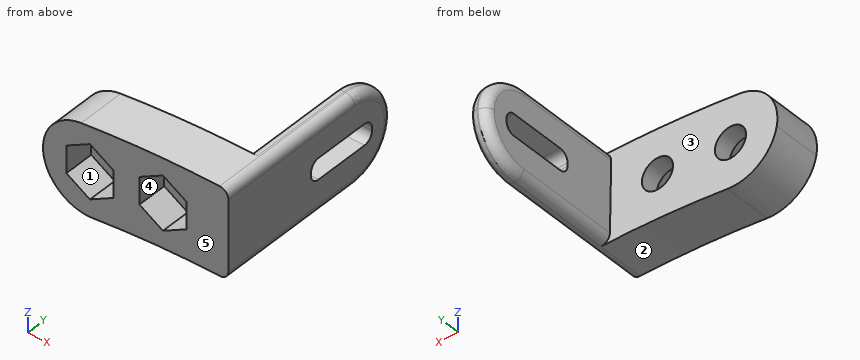
from build123d import *

# Parameters (mm, degrees)
EXTRUDE_1_DEPTH     = 8
EXTRUDE_2_DEPTH     = 25
HOLE_WIZARD_M5_1_D  = 5.3
FILLET_1_R          = 7.5
FILLET_2_DEPTH      = 8
SKETCH_5_W          = 3.5999999999999943
SKETCH_5_H          = 12.29999999986595
FILLET_3_R          = 1.5
FILLET_4_R          = 1.5
CUT_EXTRUDE_1_DEPTH = 5


with BuildPart() as part:
    # 草图1 → 凸台-拉伸1 (new body)
    with BuildSketch(Plane(origin=(0, 0, 0), x_dir=(1, 0, 0), z_dir=(0, 1, 0))):
        with BuildLine():
            Line((2.098e-14, -189), (1.932e-14, -174.00000000000003))
            ThreePointArc((2.28618e-12, -174.00000000000003), (-15.165099238093463, -173.33787746796366), (-30.214782914050144, -171.35654902412347))
            Line((-30.214782914045937, -171.35654902412418), (-32.8195055790499, -186.12866531930732))
            ThreePointArc((-32.81950557905, -186.12866531930732), (-16.472435379307413, -188.28079793933995), (-3.472e-14, -189.00000000000003))
        make_face()
    extrude(amount=EXTRUDE_1_DEPTH)

    # 草图4 → 凸台-拉伸2 (add)
    with BuildSketch(Plane(origin=(0, 8, 0), x_dir=(1, 0, 0), z_dir=(0, 1, 0))):
        with BuildLine():
            Line((2.082e-14, -189), (1.916e-14, -174))
            ThreePointArc((-3.196e-14, -174.00000000000003), (-1.5184171767173116, -173.99337461316583), (-3.0367187200877925, -173.9734989572121))
            Line((-3.036718720087315, -173.97349895721206), (-3.298504816646567, -188.97121438455795))
            ThreePointArc((-3.2985048166465822, -188.971214384558), (-1.6493152091926062, -188.99280345912842), (-3.472e-14, -189.00000000000006))
        make_face()
    extrude(amount=EXTRUDE_2_DEPTH)

    # M5 间隙孔1 (through all)
    with Locations(Plane(origin=(0, 8, 0), x_dir=(1, 0, 0), z_dir=(0, 1, 0))):
        with Locations((-23.608051681, -179.958078162), (-11.163314825, -181.156370029)):
            Hole(HOLE_WIZARD_M5_1_D / 2)

    # 圆角1
    # the kernel refuses this fillet: 7.5 mm, written as the material it takes off along each edge
    with BuildSketch(Plane(origin=(1.47232e-12, 33, -1.0760459e-10), x_dir=(0.10755019962978496, 0, 0.9941996552803635), z_dir=(0.9941996552803635, 0, -0.10755019962978496))) as fillet_1_piece_1:
        with BuildLine():
            CenterArc((174.00000000010766 + FILLET_1_R, FILLET_1_R), FILLET_1_R, 180, 89.99999999999977)
            Line((174.00000000010766 + FILLET_1_R, 0), (174.00000000010766, 0))
            Line((174.00000000010766, 0), (174.00000000010766, FILLET_1_R))
        make_face()
    fillet_1_piece_1_solid = revolve(axis=Axis((1.47232e-12, 33, -1.0760459e-10), (0, -1, 0)), revolution_arc=13.348228955549553, mode=Mode.PRIVATE)
    with BuildSketch(Plane(origin=(2.05469e-12, 33, -2.9481839e-10), x_dir=(-0.11639521392683701, 0, 0.9932029773288671), z_dir=(-0.9932029773288671, 0, -0.11639521392683701))) as fillet_1_piece_2:
        with BuildLine():
            CenterArc((189.0000000002949 - FILLET_1_R, -FILLET_1_R), FILLET_1_R, 0, 89.99999999999957)
            Line((189.0000000002949 - FILLET_1_R, 0), (189.0000000002949, 0))
            Line((189.0000000002949, 0), (189.00000000029488, -FILLET_1_R))
        make_face()
    fillet_1_piece_2_solid = revolve(axis=Axis((2.05469e-12, 33, -2.9481839e-10), (0, 1, 0)), revolution_arc=12.368210784462358, mode=Mode.PRIVATE)
    add([fillet_1_piece_1_solid, fillet_1_piece_2_solid], mode=Mode.SUBTRACT)

    # 圆角2: read off the stored shape, not the designer's step
    # 圆角2 outline → 圆角2 (cut)
    with BuildSketch(Plane(origin=(0, 0, 0), x_dir=(1, 0, 0), z_dir=(0, 1, 0))):
        with BuildLine():
            ThreePointArc((-32.819505579, -186.128665319), (-28.966041771, -186.767150281), (-25.100206236, -187.325864863))
            add(Edge.make_bspline(
                [(-25.100206236, -187.325864863), (-27.006863278382305, -187.07038767754574), (-29.132080374521447, -186.17341393049847), (-31.048536919413714, -184.35464406978926), (-32.02623112721157, -181.62978297542463), (-31.490224503, -178.589937725)],
                knots=[0, 0, 0, 0, 0, 0, 0.5103349834155644, 0.5103349834155644, 0.5103349834155644, 0.5103349834155644, 0.5103349834155644, 0.5103349834155644], degree=5, weights=[1, 0.7958660065557144, 0.6438203721908997, 0.5438630969055563, 0.4959941806996843, 0.5002136235732837]))
            Line((-31.490224503, -178.589937725), (-32.819505579, -186.128665319))
        make_face()
        with BuildLine():
            Line((-30.214782914, -171.356549024), (-31.490224503, -178.589937725))
            add(Edge.make_bspline(
                [(-31.490224503, -178.589937725), (-30.984360135627078, -175.72103774319677), (-29.29551148466263, -173.58668082656104), (-27.075163325391554, -172.48015181385665), (-24.918748626576246, -172.21612345785414), (-23.108126376, -172.458732732)],
                knots=[0.5103349834155644, 0.5103349834155644, 0.5103349834155644, 0.5103349834155644, 0.5103349834155644, 0.5103349834155644, 1, 1, 1, 1, 1, 1], degree=5, weights=[0.5002136235732837, 0.5042621674352976, 0.5562650770089762, 0.6562223522943196, 0.8041339932913276, 1]))
            ThreePointArc((-23.108126376, -172.458732732), (-26.667149567, -171.944360576), (-30.214782914, -171.356549024))
        make_face()
    extrude(amount=FILLET_2_DEPTH, mode=Mode.SUBTRACT)

    # 草图5 → 切除-旋转1 (revolve, cut)
    with BuildSketch(Plane(origin=(0, 0, 0), x_dir=(-0.01745240643728342, 0, 0.9998476951563913), z_dir=(-0.9998476951563913, 0, -0.01745240643728342))):
        with Locations((181.5, 22.85000000006228)):
            Rectangle(SKETCH_5_W, SKETCH_5_H)
    revolve(axis=Axis((0, 55.00000000000001, 0), (0, -1, 0)), mode=Mode.SUBTRACT)

    # 圆角3
    fillet_3_edges = [part.edges().sort_by_distance(p)[0] for p in [
        (-1.5995739568519802, 28.999999999995254, 183.2930204976626),
        (-1.5995739568519802, 16.700000000129307, 183.2930204976626),
        (-1.5681584290578334, 16.700000000129307, 179.6931575746316),
        (-1.5681584290578334, 28.999999999995254, 179.6931575746316),
    ]]
    fillet(fillet_3_edges, radius=FILLET_3_R)

    # 圆角4
    fillet_4_edges = [part.edges().sort_by_distance(p)[0] for p in [
        (-8.43e-15, 12.75, 189.00000000000003),
        (-3.2985048166465747, 16.75, 188.97121438455798),
        (-3.0367187200875536, 16.75, 173.9734989572121),
        (7.049e-13, 12.75, 174.00000000000003),
        (-1.5838661929561955, 33, 181.4930890361471),
        (-1.5838661929561955, 33, 181.4930890361471),
    ]]
    fillet(fillet_4_edges, radius=FILLET_4_R)

    # 草图6 → 切除-拉伸1 (cut)
    with BuildSketch(Plane.XZ):
        Polygon((-23.608051681342314, 175.33927600862347), (-19.608051681342303, 177.648677085382), (-19.608051681342303, 182.267479238899), (-23.608051681342307, 184.5768803156575), (-27.608051681342282, 182.267479238899), (-27.608051681342282, 177.64867708538196), align=None)
        Polygon((-11.163314825368905, 176.53756787555398), (-7.163314825368916, 178.84696895231247), (-7.163314825368916, 183.4657711058294), (-11.163314825368891, 185.7751721825879), (-15.16331482536884, 183.46577110582942), (-15.16331482536884, 178.84696895231244), align=None)
    extrude(amount=-CUT_EXTRUDE_1_DEPTH, mode=Mode.SUBTRACT)


solid = part.part
Source: CAD feature listing. Evaluate the final solid. Frame: model axes, mm. Face numbers are marked on the shaded views. A direction names the side the tool comes from. Round coordinates to 2 decimals unless told otherwise and drop trailing zeros. Loops run counter-clockwise (first coordinate to the right, second up) from the corner with the lowest first, then second, coordinate; pieces in that order, holes last. Notation, with made-up numbers: (-32, 3.5) - (8, 3.5) arc R13 cw to (8, 23.5) - close; hole circle Ø7 at (10.5, 79.25). An arc over 180 degrees is marked (long way). Write item = value, one per line. Start each with the question number.
(1) Section query C-C, the plane y = 14.5. Output: boundary loops of the cut face in (x, z).
(2) Set-up query: the marked faces 4 and 5. Return all of +Z, -Z, +X, -X, +Y, -Y with unobstructed straight access to the full face (end or side cutting, diameter ignored); none if empty.
(3) Section query B-B, the plane x = -10. Output: boundary loops of the cut face in (y, z).
(4) Section query A-A, the plane y = 21.5. Output: boundary loops of the cut face in (x, z).
(5) Pin query (flat end, axial travel): pin 1 (0.5 mm diameter, centred on x = -2, z = 181.5, fed in from +Y); pin 2 (5 mm diameter, centred on x = -4.5, z = 176, fed in from +Y); pin 3 (3 mm diameter, centred on x = -11.16, z = 181.16, fed in from -Y); pin 4 (4 mm diameter, centred on y = 28.5, z = 177, fed in from -X). Return the tip coordinate at first contact, or that it passes through.
(6) Pull-direction query (X, two-part tool) for the marked faces 1, 2 and 3; classes: +X half, -X half, draft (parallel to the pull), parting line (faces both ways), or undercut.
(7) Section query D-D, the plane x = -20.5. Output: boundary loops of the cut face in (y, z), plus the area to 3 significant figures.
(8) Ray query, line 1 along X through (y, z) = (4, 184.5); line 2 along X through (y, z) = (18.5, 176); line 3 along Y through (x, z) = (-6.5, 184.25). Return the intervals inside material, ascending. Write a range as from..to.
Conclusion:
q1.outline = (-3.27, 187.47) - (-3.06, 175.47) arc R1.5 ccw to (-1.55, 173.99) arc R174 cw to (-1.49, 173.99) arc R1.5 ccw to (0, 175.49) - (0, 187.49) arc R1.5 ccw to (-1.51, 188.99) arc R189 ccw to (-1.79, 188.99) arc R1.5 ccw to start
q2.face_4 = -Y
q2.face_5 = +Z, -Z, +X, -X, -Y
q3.outline = (0, 173.71) - (8, 173.71) - (8, 178.78) - (5, 178.78) - (5, 177.21) - (0, 177.21) - close; (0, 185.1) - (5, 185.1) - (5, 183.54) - (8, 183.54) - (8, 188.74) - (0, 188.74) - close
q4.outline = (-3.27, 187.47) - (-3.2, 183.27) arc R183.3 cw to (0, 183.3) - (0, 187.49) arc R1.5 ccw to (-1.51, 188.99) arc R189 ccw to (-1.79, 188.99) arc R1.5 ccw to start; (-3.14, 179.67) - (-3.06, 175.47) arc R1.5 ccw to (-1.55, 173.99) arc R174 cw to (-1.49, 173.99) arc R1.5 ccw to (0, 175.49) - (0, 179.7) arc R179.7 ccw to start
q5.pin_1 = 33
q5.pin_2 = 31.5
q5.pin_3 = through
q5.pin_4 = -3.12
q6.face_1 = undercut
q6.face_2 = +X half
q6.face_3 = draft
q7.outline = (0, 172.79) - (8, 172.79) - (8, 187.88) - (0, 187.88) - (0, 182.78) - (5, 182.78) - (5, 177.13) - (0, 177.13) - close
q7.area = 92.5 mm2
q8.line_1 = -30.02..-23.74, -23.47..-13.37, -8.95..0
q8.line_2 = -3.07..0
q8.line_3 = 0..8
